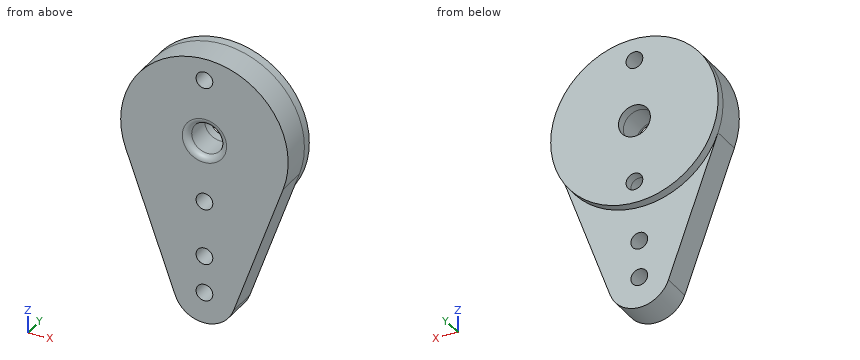
Autodesk Inventor part; units mm, degrees
ref_plane "YZ Plane" through (0, 0, 0) normal (1, 0, 0) x (0, 1, 0)
ref_plane "XZ Plane" through (0, 0, 0) normal (0, 1, 0) x (-1, 0, 0)
ref_plane "XY Plane" through (0, 0, 0) normal (0, 0, 1) x (1, 0, 0)
sketch "Boceto1" plane through (0, 0, 0) normal (0, 1, 0) x (-1, 0, 0)
  circle A0 centre (0, 0) radius 27
  circle A1 centre (0, -50) radius 10
  circle A2 centre (0, 0) radius 5.15
  line L0 (25.3915, -9.18) -> (9.4043, -53.4)
  line L1 (-25.3915, -9.18) -> (-9.4043, -53.4)
  circle A3 centre (0, -50) radius 2.7
  circle A4 centre (0, -38) radius 2.7
  circle A5 centre (0, -20) radius 2.7
  circle A6 centre (0, 20) radius 2.7
  dimension "d0" = 10.3
  dimension "d1" = 5.4
  dimension "d2" = 5.4
  dimension "d3" = 12
  dimension "d4" = 50
  dimension "d5" = 20
  dimension "d6" = 54
  dimension "d10" = 5.4
  dimension "d11" = 5.4
  dimension "d12" = 20
  dimension "d13" = 20
extrude "Extrusión1" add sketch "Boceto1" along normal blind 10 contours A0 | A0 L0 A1 A4 L1 | A1 A4 picked at (1.999, -42.9031)
sketch "Boceto3" plane through (0, 10, 0) normal (0, 1, 0) x (1, 0, 0)
  circle A0 centre (0, 0) radius 27
  circle A1 centre (0, -20) radius 2.7
  circle A2 centre (0, 0) radius 5.15
  circle A3 centre (0, 20) radius 2.7
extrude "Extrusión2" add sketch "Boceto3" along normal blind 3
fillet "Empalme1" radius 2 1 edges at (5.15, 0, 0)
properties part number "Beam support"
Design review of the part built by this model. Coordinates are the model's own, in mm. Coordinates: 2 decimals unless noted, no trailing zeros. Loops run counter-clockwise (first coordinate to the right, second up) from the corner with the lowest first, then second, coordinate; pieces in that order, holes last. Notation, with made-up numbers: (-34, 51.25) - (-11, 51.25) arc R7 cw to (-11, 56.25) - close; hole circle Ø11 at (24.25, -8.75). An arc over 180 degrees is marked (long way). Use CSV: the item, a comma, the result in double quotes. Start each with the question number.
1) Consider section B-B on x = 0. Write out the cut boundary in (y, z), then the cut area to 3 significant figures.
2) For pin 1 Ø3 at (y, z) = (4, -35.5) entering from -X; pin 2 Ø13.5 at (x, z) = (0, 0) entering from -Y; pin 3 Ø2 at (y, z) = (2, -51) entering from -X, all flat-tipped, find the tip position at first contact; note any pin that passes through.
3) Consider section A-A on z = 0. Write out the cut boundary in (x, y).
4) Wall thickness on L1, parallel to Z at x = 0, y = 6; L2, parallel to Z at x = 0, y = 11.85; L3, parallel to X at y = 11.2, z = 0: over which ranges is each line inside the solid? List them lowest first. Write a range as from..to.
5) Consider section C-C on y = 8. Write out the cut boundary in (x, z).
6) Consider section D-D on y = 11.75. Write out the cut boundary in (x, z).
Geometry says:
1,outline,"(0, -60) - (10, -60) - (10, -52.7) - (0, -52.7) - close; (0, -47.3) - (10, -47.3) - (10, -40.7) - (0, -40.7) - close; (0, -35.3) - (10, -35.3) - (10, -27) - (13, -27) - (13, -22.7) - (0, -22.7) - close; (0, -17.3) - (13, -17.3) - (13, -5.15) - (2, -5.15) arc R2 ccw to (0, -7.15) - close; (0, 7.15) arc R2 ccw to (2, 5.15) - (13, 5.15) - (13, 17.3) - (0, 17.3) - close; (0, 22.7) - (13, 22.7) - (13, 27) - (0, 27) - close"
1,area,"648 mm^2"
2,pin 1,"x = -16.42"
2,pin 2,"y = 0.04"
2,pin 3,"x = -10.63"
3,outline,"(-27, 0) - (-7.15, 0) arc R2 ccw to (-5.15, 2) - (-5.15, 13) - (-27, 13) - close; (5.15, 2) arc R2 ccw to (7.15, 0) - (27, 0) - (27, 13) - (5.15, 13) - close"
4,L1,"-60..-52.7, -47.3..-40.7, -35.3..-22.7, -17.3..-5.15, 5.15..17.3, 22.7..27"
4,L2,"-27..-22.7, -17.3..-5.15, 5.15..17.3, 22.7..27"
4,L3,"-27..-5.15, 5.15..27"
5,outline,"(-25.39, -9.18) - (-9.4, -53.4) arc R10 ccw to (9.4, -53.4) - (25.39, -9.18) arc R27 ccw (long way) to start; hole circle Ø10.3 at (0, 0); hole circle Ø5.4 at (0, -50); hole circle Ø5.4 at (0, -38); hole circle Ø5.4 at (0, -20); hole circle Ø5.4 at (0, 20)"
6,outline,"circle Ø54 at (0, 0); hole circle Ø10.3 at (0, 0); hole circle Ø5.4 at (0, -20); hole circle Ø5.4 at (0, 20)"
